```python
from build123d import *

# Parameters (mm, degrees)
F1_DEPTH = 2.54


with BuildPart() as f1:
    # F0 (on Front) → F1 (new body)
    with BuildSketch(Plane.XZ):
        with BuildLine():
            ThreePointArc((-145.7550496822, -1.980112821), (-145.6599833362, -2.3612365902), (-145.6280121514, -2.752734714))
            ThreePointArc((-145.6280121514, -2.752734714), (-146.4936146234, -4.6042556807), (-148.4693962296, -5.1274043924))
            Line((-148.4693962296, -5.1274043924), (-187.0211775011, -218.8322330784))
            ThreePointArc((-187.0211775011, -218.8322330784), (-186.3483570952, -219.0277166776), (-185.7305923943, -219.3582736479))
            Line((-185.7305923943, -219.3582736479), (-8.4100794876, 42.2926197897))
            ThreePointArc((-8.4100794876, 42.2926197897), (-9.2000837984, 43.0403550137), (-9.7103273998, 44.0010142893))
            Line((-9.7103273998, 44.0010142893), (-145.7550496822, -1.980112821))
        make_face()
        with BuildLine():
            ThreePointArc((-3.1565113243, 45.0786185085), (-7.0680481812, 48.3995271192), (-9.7103273998, 44.0010142893))
            Line((-9.7103273998, 44.0010142893), (-6.5220113243, 45.0786185085))
            Line((-6.5220113243, 45.0786185085), (-8.4100794876, 42.2926197897))
            ThreePointArc((-8.4100794876, 42.2926197897), (-4.9452588316, 42.1053304587), (-3.1565113243, 45.0786185085))
        make_face()
        with BuildLine():
            Line((-6.5220113243, 45.0786185085), (-9.7103273998, 44.0010142893))
            ThreePointArc((-9.7103273998, 44.0010142893), (-9.2000837984, 43.0403550137), (-8.4100794876, 42.2926197897))
            Line((-8.4100794876, 42.2926197897), (-6.5220113243, 45.0786185085))
        make_face()
        with BuildLine():
            ThreePointArc((-148.4693962296, -5.1274043924), (-146.4936146234, -4.6042556807), (-145.6280121514, -2.752734714))
            ThreePointArc((-145.6280121514, -2.752734714), (-145.6599833362, -2.3612365902), (-145.7550496822, -1.980112821))
            Line((-145.7550496822, -1.980112821), (-148.0410121514, -2.752734714))
            Line((-148.0410121514, -2.752734714), (-148.4693962296, -5.1274043924))
        make_face()
        with BuildLine():
            Line((-148.0410121514, -2.752734714), (-145.7550496822, -1.980112821))
            ThreePointArc((-145.7550496822, -1.980112821), (-149.8683080849, -1.1768036966), (-148.4693962296, -5.1274043924))
            Line((-148.4693962296, -5.1274043924), (-148.0410121514, -2.752734714))
        make_face()
        with BuildLine():
            Line((-187.6186605575, -222.1442723667), (-187.0211775011, -218.8322330784))
            ThreePointArc((-187.0211775011, -218.8322330784), (-190.2010450638, -224.3024847084), (-184.2531605575, -222.1442723667))
            ThreePointArc((-184.2531605575, -222.1442723667), (-184.6453725078, -220.567519874), (-185.7305923943, -219.3582736479))
            Line((-185.7305923943, -219.3582736479), (-187.6186605575, -222.1442723667))
        make_face()
        with BuildLine():
            ThreePointArc((-185.7305923943, -219.3582736479), (-186.3483570952, -219.0277166776), (-187.0211775011, -218.8322330784))
            Line((-187.0211775011, -218.8322330784), (-187.6186605575, -222.1442723667))
            Line((-187.6186605575, -222.1442723667), (-185.7305923943, -219.3582736479))
        make_face()
    extrude(amount=F1_DEPTH)


solid = f1.part
```
Work out the finished part from the listing and answer in its coordinate system (mm). Round coordinates to 2 decimals unless told otherwise and drop trailing zeros. Write each loop counter-clockwise with the first axis right and the second up, starting at its lowest first coordinate (ties: lowest second). Pieces come first, ordered by that corner, then holes.
1) A cutting plane is placed at C-C on x = -70. Determine the outline of the cut face in (y, z), and give its area (3 significant figures).
2) Determine the mould class of faces 1 (the face through (-111, 0, -57)), 2 (the face through (-111, -2.54, -57)), 3 (the face through (-167.475, -1.252, -110.484)) for opening direction Y: pulls with the +Y half, pulls with the -Y half, needs draft (parallel to the pull), parting line crosses it, or undercut.
3) Consider probe 1 along X at (y, z) = (-0.35, -8.5); probe 2 along Z at (x, y) = (-25, -0.05); probe 3 along X at (y, z) = (-2.4, -123). Determine where each line is inside the solid, lowest interval first.
4) A cutting plane is placed at A-A on y = -0.5. Determine the outline of the cut face in (x, z), and give its area (3 significant figures).
5) A cutting plane is placed at B-B on z = -56. Determine the outline of the cut face in (x, y), and give its area (3 significant figures).
6) A flat-ended cylindrical pin translates along its axis: P1, Ø1.5, axis at y = -2, z = -106.5, coming from the +X side. Find the tip coordinate at first contact, or state that the pin passes through.
Entries:
1. outline: (-2.54, -48.59) - (0, -48.59) - (0, 23.62) - (-2.54, 23.62) - close
1. area: 183 mm2
2. face 1: pulls with the +Y half
2. face 2: pulls with the -Y half
2. face 3: needs draft
3. probe 1: x = -149.08 to -42.83
3. probe 2: z = 17.81 to 38.83
3. probe 3: x = -169.73 to -120.43
4. outline: (-187.02, -218.83) arc R3.37 ccw (long way) to (-185.73, -219.36) - (-8.41, 42.29) arc R3.37 ccw (long way) to (-9.71, 44) - (-145.76, -1.98) arc R2.41 ccw (long way) to (-148.47, -5.13) - close
4. area: 14,700 mm2
5. outline: (-157.65, -2.54) - (-75.02, -2.54) - (-75.02, 0) - (-157.65, 0) - close
5. area: 210 mm2
6. P1: stops at x = -108.74
